Design review of the part built by this model. Coordinates are the model's own, in mm. A direction names the side the tool comes from. Give positions to 0.01 mm unless a question says otherwise; leave off trailing zeros. Order: outer loops, then holes, each group sorted by start corner. A loop starts at its lowest first (then second) coordinate and runs counter-clockwise, first axis right, second up. Notation, with made-up numbers: (-35, 17.25) -> (-6, 17.25) arc R16 ccw to (-6, 23.25) -> close; hole circle Ø7 at (-26, -7.75). An arc over 180 degrees is marked (long way). One line per item, written item: value. Start each with the question number.
1) Tool access review of faces 5 (the face through (0, 0, 0)), 6 (the face through (64.4, 12.93, -4.9)), 7 (the face through (69, -14.7, 0)), 8 (the face through (61, 16.5, -2)), 9 (the face through (64, 14, -7.119)): name each direction out of +Z, -Z, +X, -X, +Y, -Y from which nothing blocks a thin tool from reaching the whole face with its end or side.
2) The part is to be moulded in two halves that separate along Y. For faces 1 (the face through (111, 0, -2.619)), 2 (the face through (-1, -4.5, 1)), 3 (the face through (68.6, 12.93, -4.9)), 4 (the face through (1.61, 13.08, -4.33)), say which applies: released by +Y, released by -Y, zero draft, split by the parting line, or undercut.
3) Consider section B-B (z = -0.5). State the section outline as (x, y) points, plus the area to 3 significant figures.
4) Wall thickness on line 1 along X through (y, z) = (-3, -5); line 2 along Y through (x, z) = (65, -1.25); line 3 along Y through (x, z) = (29, -5.25): over which ranges is each line inside the solid? List them lowest first. Write a range as from..to.
5) Consider section C-C (x = 33). State the section outline as (y, z) points, plus the area to 3 significant figures.
6) For pin 1 (1.3 mm diameter, centred on y = 3.5, z = -4, fed in from +X); pin 2 (5 mm diameter, centred on y = -9, z = -2, fed in from -X); pin 3 (6.5 mm diameter, centred on x = 113, y = -4, fed in from +Z), all flat-tipped, find the tip position at first contact; note any pin that passes through.
7) Consider section A-A (x = 95). State the section outline as (y, z) points.
from build123d import *

# Parameters (mm, degrees)
BOSS_EXTRUDE2_DEPTH                    = 5.5
SKETCH4_W                              = 3
SKETCH4_H                              = 27
BOSS_EXTRUDE4_CROSS_STRUCTURES_DEPTH   = 5.5
SKETCH6_W                              = 3
SKETCH6_H                              = 27
CUT_EXTRUDE3_1_MM_SPACING_DEPTH        = 1
CUT_EXTRUDE4_ELECTRONICS_SPACING_DEPTH = 124.233518168
SKETCH8_W                              = 5.5
SKETCH8_H                              = 14
CUT_EXTRUDE2_USB_C_CUTOUT_DEPTH        = 5
FILLET2_USBC_R                         = 2
FILLET3_INNER_CORNERS_FRONT_R          = 1
FILLET5_INNER_CORNERS_R                = 2
SKETCH18_W                             = 62
SKETCH18_H                             = 1.8
SKETCH18_W_2                           = 2
SKETCH18_H_2                           = 9
BOSS_EXTRUDE7_DEPTH                    = 5
FILLET1_R                              = 1


with BuildPart() as part:
    # Sketch3 → Boss-Extrude2 (new body)
    with BuildSketch(Plane.XY.offset(-1.6194024)):
        with BuildLine():
            Line((110, 16.5), (10, 16.5))
            ThreePointArc((10, 16.5), (1.514718626, 12.985281374), (-2, 4.5))
            Line((-2, 4.5), (-2, -4.5))
            ThreePointArc((-2, -4.5), (1.514718626, -12.985281374), (10, -16.5))
            Line((10, -16.5), (110, -16.5))
            ThreePointArc((110, -16.5), (118.485281374, -12.985281374), (122, -4.5))
            Line((122, -4.5), (122, 4.5))
            ThreePointArc((122, 4.5), (118.485281374, 12.985281374), (110, 16.5))
        make_face()
        with BuildLine():
            Line((119, -4.5), (119, 4.5))
            ThreePointArc((119, 4.5), (116.363961031, 10.863961031), (110, 13.5))
            Line((110, 13.5), (10, 13.5))
            ThreePointArc((10, 13.5), (3.636038969, 10.863961031), (1, 4.5))
            Line((1, 4.5), (1, -4.5))
            ThreePointArc((1, -4.5), (3.636038969, -10.863961031), (10, -13.5))
            Line((10, -13.5), (110, -13.5))
            ThreePointArc((110, -13.5), (116.363961031, -10.863961031), (119, -4.5))
        make_face(mode=Mode.SUBTRACT)
    extrude(amount=-BOSS_EXTRUDE2_DEPTH)

    # Sketch4 → Boss-Extrude4 - cross structures (add)
    with BuildSketch(Plane.XY.offset(-1.6194024)):
        with Locations((110.9, 0)):
            Rectangle(SKETCH4_W, SKETCH4_H)
        with Locations((66.5, 0)):
            Rectangle(SKETCH4_W, SKETCH4_H)
    extrude(amount=-BOSS_EXTRUDE4_CROSS_STRUCTURES_DEPTH)

    # Sketch6 → Cut-Extrude3 - 1 mm spacing (cut)
    with BuildSketch(Plane.XY.offset(-1.6194024)):
        with BuildLine():
            Line((109.4, 13.5), (110, 13.5))
            ThreePointArc((110, 13.5), (111.211013131, 13.418152678), (112.4, 13.174099377))
            Line((112.4, 13.174099377), (112.4, -13.174099377))
            ThreePointArc((112.4, -13.174099377), (111.211013131, -13.418152678), (110, -13.5))
            Line((110, -13.5), (109.4, -13.5))
            Line((109.4, -13.5), (109.4, 13.5))
        make_face()
        with Locations((66.5, 0)):
            Rectangle(SKETCH6_W, SKETCH6_H)
    extrude(amount=-CUT_EXTRUDE3_1_MM_SPACING_DEPTH, mode=Mode.SUBTRACT)

    # Sketch7 → Cut-Extrude4 - electronics spacing (cut, through all)
    with BuildSketch(Plane.XY.offset(-1.6194024)):
        with BuildLine():
            Line((38, -14.5), (10, -14.5))
            ThreePointArc((10, -14.5), (8.99491038, -14.44936153), (8, -14.297958971))
            Line((8, -14.297958971), (8, 14.297958971))
            ThreePointArc((8, 14.297958971), (8.99491038, 14.44936153), (10, 14.5))
            Line((10, 14.5), (38, 14.5))
            Line((38, 14.5), (38, -14.5))
        make_face()
    extrude(amount=-CUT_EXTRUDE4_ELECTRONICS_SPACING_DEPTH, mode=Mode.SUBTRACT)

    # Sketch8 → Cut-Extrude2 - USB-C cutout (cut)
    with BuildSketch(Plane(origin=(122, 0, 0), x_dir=(0, 0, -1), z_dir=(1, 0, 0))):
        with Locations((4.3694024, 0)):
            Rectangle(SKETCH8_W, SKETCH8_H)
    extrude(amount=-CUT_EXTRUDE2_USB_C_CUTOUT_DEPTH, mode=Mode.SUBTRACT)

    # Fillet2 - USBC
    fillet2_usbc_edges = [part.edges().sort_by_distance(p)[0] for p in [
        (120.191251414, 7, -7.1194024),
        (120.191251414, -7, -7.1194024),
    ]]
    fillet(fillet2_usbc_edges, radius=FILLET2_USBC_R)

    # Fillet3 - inner corners, front
    fillet3_inner_corners_front_edges = [part.edges().sort_by_distance(p)[0] for p in [
        (38, 13.5, -4.3694024),
        (38, -13.5, -4.3694024),
        (8, -13.274964387, -4.3694024),
        (8, 13.274964387, -4.3694024),
    ]]
    fillet(fillet3_inner_corners_front_edges, radius=FILLET3_INNER_CORNERS_FRONT_R - 0.0001)  # a hair under: the kernel refuses the full size

    # Fillet5 - inner corners
    fillet5_inner_corners_edges = [part.edges().sort_by_distance(p)[0] for p in [
        (112.4, -13.174099377, -4.8694024),
        (109.4, -13.5, -4.8694024),
        (109.4, 13.5, -4.8694024),
        (65, -13.5, -4.8694024),
        (65, 13.5, -4.8694024),
        (68, 13.5, -4.8694024),
        (68, -13.5, -4.8694024),
        (112.4, 13.174099377, -4.8694024),
    ]]
    fillet(fillet5_inner_corners_edges, radius=FILLET5_INNER_CORNERS_R)

    # Sketch18 → Boss-Extrude7 (add)
    with BuildSketch(Plane.XY.offset(-1.6194024)):
        with Locations((69, 15.6)):
            Rectangle(SKETCH18_W, SKETCH18_H)
        with Locations((69, -15.6)):
            Rectangle(SKETCH18_W, SKETCH18_H)
        with Locations((-1, 0)):
            Rectangle(SKETCH18_W_2, SKETCH18_H_2)
    extrude(amount=BOSS_EXTRUDE7_DEPTH)

    # Fillet1
    fillet1_edges = [part.edges().sort_by_distance(p)[0] for p in [
        (69, 14.7, 3.3805976),
        (69, -14.7, 3.3805976),
        (0, 0, 3.3805976),
    ]]
    fillet(fillet1_edges, radius=FILLET1_R)


solid = part.part
Checked values:
1. face 5: +Z, +X, +Y, -Y
1. face 6: +Z, -Z
1. face 7: +Z, +X, -X
1. face 8: +Z, -Z, +X, -X, +Y
1. face 9: -Z, +X, -X, +Y, -Y
2. face 1: undercut
2. face 2: released by -Y
2. face 3: undercut
2. face 4: released by +Y
3. outline: (-2, -4.5) -> (0, -4.5) -> (0, 4.5) -> (-2, 4.5) -> close; (38, -16.5) -> (100, -16.5) -> (100, -14.7) -> (38, -14.7) -> close; (38, 14.7) -> (100, 14.7) -> (100, 16.5) -> (38, 16.5) -> close
3. area: 241 mm^2
4. line 1: x = -2..1, 65..68, 109.4..112.4
4. line 2: y = -16.5..-14.7, 14.7..16.5
4. line 3: y = -16.5..-14.5, 14.5..16.5
5. outline: (-16.5, -7.12) -> (-14.5, -7.12) -> (-14.5, -1.62) -> (-16.5, -1.62) -> close; (14.5, -7.12) -> (16.5, -7.12) -> (16.5, -1.62) -> (14.5, -1.62) -> close
5. area: 22.0 mm^2
6. pin 1: stops at x = 112.4
6. pin 2: stops at x = -1.83
6. pin 3: stops at z = -2.62
7. outline: (-16.5, -7.12) -> (-13.5, -7.12) -> (-13.5, -1.62) -> (-14.7, -1.62) -> (-14.7, 2.38) arc R1 ccw to (-15.7, 3.38) -> (-16.5, 3.38) -> close; (13.5, -7.12) -> (16.5, -7.12) -> (16.5, 3.38) -> (15.7, 3.38) arc R1 ccw to (14.7, 2.38) -> (14.7, -1.62) -> (13.5, -1.62) -> close
